Autodesk Inventor part; units mm, degrees
ref_plane "작업 평면1" through (0, 0, -56.25) normal (0, 0, 1) x (1, 0, 0)
ref_plane "YZ Plane" through (0, 0, 0) normal (1, 0, 0) x (0, 1, 0)
ref_plane "XZ Plane" through (0, 0, 0) normal (0, 1, 0) x (-1, 0, 0)
sketch "스케치1" plane through (0, 0, 0) normal (0, 0, 1) x (1, 0, 0)
  line L0 (-7.5, -15) -> (7.5, -15)
  line L1 (7.5, -15) -> (7.5, 15)
  line L2 (7.5, 15) -> (-7.5, 15)
  line L3 (-7.5, 15) -> (-7.5, -15)
  point P0 (0, 0)
  dimension "d0" = 15
  dimension "d1" = 30
  dimension "d2" = 15
  dimension "d3" = 7.5
extrude "돌출1" add sketch "스케치1" against normal blind 37.5
sketch "스케치2" plane through (0, 0, -37.5) normal (0, 0, -1) x (-1, 0, 0)
  line L0 (5, 11.25) -> (-5, 11.25)
  line L1 (-5, 11.25) -> (-5, -11.25)
  line L2 (-5, -11.25) -> (5, -11.25)
  line L3 (5, -11.25) -> (5, 11.25)
  line L4 (5, 11.25) -> (-5, -11.25) construction
  line L5 (-5, 11.25) -> (5, -11.25) construction
  line L6 (-4, -10) -> (4, -10)
  line L7 (4, -10) -> (4, 10)
  line L8 (4, 10) -> (-4, 10)
  line L9 (-4, 10) -> (-4, -10)
  line L10 (-4, -10) -> (4, 10) construction
  line L11 (4, -10) -> (-4, 10) construction
  point P0 (0, 0)
  dimension "d6" = 10
  dimension "d7" = 22.5
  dimension "d10" = 8
  dimension "d11" = 20
extrude "돌출2" add sketch "스케치2" along normal blind 75
sketch "스케치3" plane through (0, 0, 0) normal (0, 0, 1) x (1, 0, 0)
  line L0 (-3.95, -5) -> (3.95, -5)
  line L1 (3.95, -5) -> (3.95, 5)
  line L2 (3.95, 5) -> (-3.95, 5)
  line L3 (-3.95, 5) -> (-3.95, -5)
  line L4 (-3.95, -5) -> (3.95, 5) construction
  line L5 (3.95, -5) -> (-3.95, 5) construction
  point P0 (0, 0)
  dimension "d12" = 7.9
  dimension "d13" = 10
extrude "돌출3" add sketch "스케치3" along normal blind 15
sketch "스케치4" plane through (3.95, -5, 0) normal (1, 0, 0) x (0, 0, -1)
  circle A0 centre (-10, 5) radius 2.1
  line L0 (0, 0) -> (-15, 0)
  line L1 (-15, 0) -> (-15, 10)
  point P0 (0, 5)
  dimension "d16" = 4.2
  dimension "d17" = 5
  dimension "d18" = 5
extrude "돌출4" cut sketch "스케치4" against normal blind 15
sketch "스케치5" plane through (0, 0, -112.5) normal (0, 0, -1) x (-1, 0, 0)
  line L0 (-5, 11.25) -> (5, 11.25)
  line L1 (5, -11.25) -> (-5, -11.25)
  line L2 (5, 11.25) -> (-5, 11.25)
  line L3 (-5, 11.25) -> (-5, -11.25)
  line L4 (-5, -11.25) -> (5, -11.25)
  line L5 (5, -11.25) -> (5, 11.25)
  point P0 (7.5, 15)
  point P1 (-7.5, -15)
extrude "돌출5" add sketch "스케치5" against normal blind 2
ref_plane "작업 평면1" through (0, 0, -56.25) normal (0, 0, 1) x (1, 0, 0)
mirror "미러1" about plane through (0, 0, -56.25) normal (0, 0, 1) of "돌출3"
mirror "미러2" about plane through (0, 0, -56.25) normal (0, 0, 1) of "돌출4"
fillet "모깎기1" radius 4 4 edges at (0, -5, 15) (0, 5, 15) (0, -5, -127.5) (0, 5, -127.5)
properties part number "각도조절 액추에이터_중간" material "스테인리스스틸"
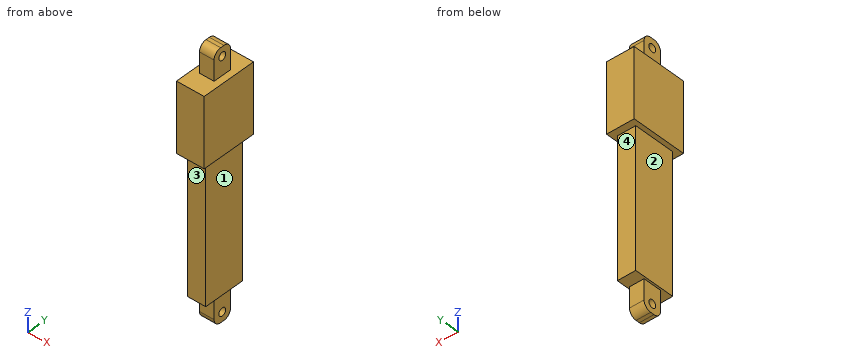
Part model, mm, in its own coordinate system. Face numbers are marked on the shaded views. A direction names the side the tool comes from. Give positions to 0.01 mm unless a question says otherwise; leave off trailing zeros. Write each loop counter-clockwise with the first axis right and the second up, starting at its lowest first coordinate (ties: lowest second). Pieces come first, ordered by that corner, then holes. Notation, with made-up numbers: (89.25, 20) -> (132.25, 20) arc R24 cw to (132.25, 32) -> close; hole circle Ø7 at (70, 79). An arc over 180 degrees is marked (long way). Put each result on its own line as item: value. Start each with the question number.
Item 1: Cut at B-B (z = -94.5). List the corners of the cut face in (x, y), then the cut area to 3 significant figures.
Item 2: Cut at A-A (y = 6.25). List the corners of the cut face in (x, z), then the cut area to 4 significant figures.
Item 3: Pin check, flat tips, straight feed: pin 1 Ø4 at (x, z) = (1, 4) entering from +Y; pin 2 Ø5 at (x, y) = (2.5, -8) entering from +Z; pin 3 Ø4 at (x, z) = (-2, -112.5) entering from +Y; pin 4 Ø11 at (y, z) = (-2, 4) entering from -X. Stop position of each tip, or through.
Item 4: Which spindle directions (+Z, -Z, +X, -X, +Y, -Y) get a long thin tool onto all of the face, cutting with end or side? Do the marked faces 1, 2, 3 and 4. Say none if no direction does.
Item 5: Wall check: L1, parallel to Z at x = 1, y = 0.25; L2, parallel to X at y = -2.5, z = -68.5; L3, parallel to Y at x = -2, z = 10. Give the ranges that are in metal, low to high. Write a range as [from, to].
Answer list:
1. outline: (-5, -11.25) -> (5, -11.25) -> (5, 11.25) -> (-5, 11.25) -> close; hole (-4, -10) -> (4, -10) -> (4, 10) -> (-4, 10) -> close
1. area: 65.0 mm2
2. outline: (-7.5, -37.5) -> (-5, -37.5) -> (-5, -112.5) -> (5, -112.5) -> (5, -37.5) -> (7.5, -37.5) -> (7.5, 0) -> (-7.5, 0) -> close; hole (-4, -110.5) -> (4, -110.5) -> (4, -37.5) -> (-4, -37.5) -> close
2. area: 728.5 mm2
3. pin 1: stops at y = 5
3. pin 2: stops at z = 0
3. pin 3: stops at y = 11.25
3. pin 4: stops at x = -7.5
4. face 1: -Z, +X, +Y, -Y
4. face 2: -Z, -X, +Y, -Y
4. face 3: -Z, +X, -X, -Y
4. face 4: -Z, +X, -X, +Y
5. L1: z = [-127.5, -124.59], [-120.41, -110.5], [-37.5, 7.91], [12.09, 15]
5. L2: x = [-5, -4], [4, 5]
5. L3: y = [-5, -2.1], [2.1, 5]
